Geometry check sheet. Reference: the model listing, model coordinates, mm. A direction names the side the tool comes from. Coordinates: 2 decimals unless noted, no trailing zeros. Loops run counter-clockwise (first coordinate to the right, second up) from the corner with the lowest first, then second, coordinate; pieces in that order, holes last. Notation, with made-up numbers: (17.25, 3.25) -> (51.25, 3.25) arc R25 cw to (51.25, 35.25) -> close; hole circle Ø11 at (26, 10). An arc over 180 degrees is marked (long way). Answer as a JSON object with one key per item and string values.
from build123d import *

# Parameters (mm, degrees)
PAD_DEPTH            = 16
SKETCH002_R          = 4
PAD001_DEPTH         = 0.85
SKETCH003_R          = 4
PAD002_DEPTH         = 0.85
SKETCH004_R          = 2.5
POCKET001_DEPTH      = 32.001
CHAMFER_SIZE         = 0.84
CHAMFER020021_SIZE   = 0.4
CHAMFER020022_SIZE   = 3
CHAMFER020023_SIZE   = 8
SKETCH005_R          = 1.55
POCKET_DEPTH         = 16.001
SKETCH006_R          = 1.9
POCKET002_DEPTH      = 7
CHAMFER020024_SIZE   = 0.4
BODY_PLACEMENT_ANGLE = 270


with BuildPart() as part:
    # Sketch → Pad (new body)
    with BuildSketch(Plane.YZ):
        Polygon((-8.85, 6), (8, 6), (8, -6), (-8.85, -6), (-8.85, -11.85), (8.15, -11.85), (8.15, -20), (18, -20), (18, 20), (8.15, 20), (8.15, 11.85), (-8.85, 11.85), align=None)
    extrude(amount=PAD_DEPTH)

    # Sketch002 (on DatumPlane) → Pad001 (join)
    with BuildSketch(Plane.XY.offset(-6)):
        with Locations((8, 0)):
            Circle(SKETCH002_R)
    extrude(amount=PAD001_DEPTH)

    # Sketch003 (on DatumPlane) → Pad002 (join)
    with BuildSketch(Plane.XY.offset(6)):
        with Locations((8, 0)):
            Circle(SKETCH003_R)
    extrude(amount=-PAD002_DEPTH)

    # Sketch004 (on DatumPlane) → Pocket001 (cut, through all)
    with BuildSketch(Plane.XY.offset(-12)):
        with Locations((8, 0)):
            Circle(SKETCH004_R)
    extrude(amount=POCKET001_DEPTH, mode=Mode.SUBTRACT)

    # Chamfer
    chamfer_edges = [part.edges().sort_by_distance(p)[0] for p in [
        (4, 0, -5.15),
        (4, 0, 5.15),
    ]]
    chamfer(chamfer_edges, length=CHAMFER_SIZE)

    # Chamfer020021
    chamfer020021_edges = [part.edges().sort_by_distance(p)[0] for p in [
        (5.5, 0, -11.85),
        (5.5, 0, 11.85),
    ]]
    chamfer(chamfer020021_edges, length=CHAMFER020021_SIZE)

    # Chamfer020022
    chamfer020022_edges = [part.edges().sort_by_distance(p)[0] for p in [
        (0, -8.85, 8.925),
        (16, -8.85, 8.925),
        (0, -8.85, -8.925),
        (16, -8.85, -8.925),
    ]]
    chamfer(chamfer020022_edges, length=CHAMFER020022_SIZE)

    # Chamfer020023
    chamfer020023_edges = [part.edges().sort_by_distance(p)[0] for p in [
        (8, 18, 20),
        (8, 18, -20),
    ]]
    chamfer(chamfer020023_edges, length=CHAMFER020023_SIZE)

    # Sketch005 (on DatumPlane) → Pocket (cut, through all)
    with BuildSketch(Plane.YZ.offset(16)):
        with Locations((13, 0)):
            Circle(SKETCH005_R)
    extrude(amount=-POCKET_DEPTH, mode=Mode.SUBTRACT)

    # Sketch006 (on DatumPlane) → Pocket002 (cut)
    with BuildSketch(Plane.YZ):
        with Locations((13, 0)):
            Circle(SKETCH006_R)
    extrude(amount=POCKET002_DEPTH, mode=Mode.SUBTRACT)

    # Chamfer020024
    chamfer020024_edges = [part.edges().sort_by_distance(p)[0] for p in [
        (16, 1.15, 11.85),
        (16, 8.15, 15.925),
        (16, 9.075, 20),
        (16, 14, 16),
        (16, 11.45, 0),
        (16, 14, -16),
        (16, 18, 0),
        (16, 8.15, -15.925),
        (16, 9.075, -20),
        (16, 1.15, -11.85),
        (16, 1.075, -6),
        (14.5, -7.35, -6),
        (14.5, -7.35, -11.85),
        (8, -8.85, -6),
        (8, -8.85, -11.85),
        (0, 8.15, -15.925),
        (0, 1.15, -11.85),
        (1.5, -7.35, -11.85),
        (1.5, -7.35, -6),
        (0, 1.075, -6),
        (0, 9.075, -20),
        (0, 14, -16),
        (0, 18, 0),
        (0, 11.1, 0),
        (0, 14, 16),
        (0, 9.075, 20),
        (0, 8.15, 15.925),
        (0, 1.15, 11.85),
        (0, 8, 0),
        (0, 1.075, 6),
        (1.5, -7.35, 6),
        (1.5, -7.35, 11.85),
        (8, -8.85, 11.85),
        (8, -8.85, 6),
        (14.5, -7.35, 6),
        (16, 1.075, 6),
        (16, 8, 0),
        (8, 8.15, -20),
        (8, 8.15, 20),
        (14.5, -7.35, 11.85),
    ]]
    chamfer(chamfer020024_edges, length=CHAMFER020024_SIZE)


with BuildPart() as part_1:
    # Body placement: moved
    add(part.part.moved(Location((9, 0, 14))).rotate(Axis((9, 0, 14), (0, 0, 1)), BODY_PLACEMENT_ANGLE))


solid = part_1.part
1. Section check B-B, the plane x = 15. Record the boundary of the cut face in (y, z), then the cut area to 3 significant figures.
Evaluation:
{"outline": "(-16, 2.55) -> (-15.6, 2.15) -> (-0.4, 2.15) -> (0, 2.55) -> (0, 7.6) -> (-0.4, 8) -> (-15.6, 8) -> (-16, 7.6) -> close; (-16, 20.4) -> (-15.6, 20) -> (-0.4, 20) -> (0, 20.4) -> (0, 25.45) -> (-0.4, 25.85) -> (-15.6, 25.85) -> (-16, 25.45) -> close", "area": "187 mm^2"}
2. Depth check by flat-ended pin: P1, Ø8, axis at x = 9, y = -8, coming from the -Z side; P2, Ø6, axis at y = -5.5, z = 28.5, coming from the -X side; P3, Ø8, axis at y = -5.5, z = 14.5, coming from the -X side. Enter the tip coordinate at first touch or a pass-through.
Evaluation:
{"P1": "stops at z = 2.15", "P2": "stops at x = 0.2", "P3": "stops at x = 17"}
3. Section check D-D, the plane z = 14. Record the boundary of the cut face in (x, y).
Evaluation:
{"outline": "(17, -15.6) -> (17.4, -16) -> (20.05, -16) -> (20.45, -15.6) -> (20.45, -7) -> (20.1, -7) -> (20.1, -0.4) -> (19.7, 0) -> (17.4, 0) -> (17, -0.4) -> close; (23.55, -15.6) -> (23.95, -16) -> (26.6, -16) -> (27, -15.6) -> (27, -0.4) -> (26.6, 0) -> (24.3, 0) -> (23.9, -0.4) -> (23.9, -7) -> (23.55, -7) -> close"}
4. Section check A-A, the plane z = 4. Record the boundary of the cut face in (x, y).
Evaluation:
{"outline": "(0.15, -13) -> (3.15, -16) -> (26.6, -16) -> (27, -15.6) -> (27, -0.4) -> (26.6, 0) -> (3.15, 0) -> (0.15, -3) -> close; hole circle Ø5 at (9, -8)"}
5. Section check C-C, the plane y = -8. State how many separate pieces and enclosed holes the cut face has, then the cut area to 3 significant figures.
Evaluation:
{"separate pieces": "3", "enclosed holes": "1", "area": "468 mm^2"}
6. Mould release check, pull along Y, two halves, no side actions. Record for faces 1 (the face through (6.78, -9.15, 5.66)), 2 (the face through (1.81, -1.62, 7.8)), 3 (the face through (22.913, -15.803, -1.801)): released by +Y, released by -Y, zero draft, split by the parting line, or undercut.
Evaluation:
{"face 1": "undercut", "face 2": "released by +Y", "face 3": "released by -Y"}
7. Tool access check on faces 4 (the face through (17.15, -8, 30)), 5 (the face through (20.1, -3.65, 14.08)), 6 (the face through (8.7, -4.5, 2.15)). Record the directions out of +Z, -Z, +X, -X, +Y, -Y that give a thin tool (end or side, any length) a straight path to the whole face; none if there is none.
Evaluation:
{"face 4": "+Z, -X, +Y, -Y", "face 5": "+Y", "face 6": "-Z, -X, +Y, -Y"}
8. Thickness scan on probe 1 along X at (y, z) = (-8, 24.25); probe 2 along Z at (x, y) = (7.75, -0.75); probe 3 along Y at (x, z) = (9, 5.5). Record the ranges inside material, lowest first. Write a range as from..to.
Evaluation:
{"probe 1": "x = 0.15..6.5, 11.5..27", "probe 2": "z = 2.15..8, 20..25.85", "probe 3": "y = -16..-10.5, -5.5..0"}
